from build123d import *

# Parameters (mm, degrees)
SKETCH1_R                = 1.5
SKETCH1_R_2              = 2.5
BOSS_EXTRUDE1_DEPTH      = 20
SKETCH2_W                = 8.1
SKETCH2_H                = 20
SKETCH2_W_2              = 5.2
SKETCH2_W_3              = 5.1
CUT_EXTRUDE1_DEPTH       = 20
CUT_EXTRUDE1_DEPTH_BACK  = 20
CUT_EXTRUDE2_DEPTH       = 9
BOSS_EXTRUDE2_DEPTH      = 11.9
SKETCH5_R                = 3
BOSS_EXTRUDE3_DEPTH      = 5
CUT_EXTRUDE6_DEPTH       = 1
SKETCH13_R               = 2.5
CUT_EXTRUDE7_DEPTH       = 4
BOSS_EXTRUDE4_DEPTH      = 3
CUT_EXTRUDE9_DEPTH       = 3
SKETCH17_W               = 9
SKETCH17_H               = 3.569322199
CUT_EXTRUDE11_DEPTH      = 3
SKETCH18_W               = 5.770974844
SKETCH18_H               = 0.772936936
BOSS_EXTRUDE5_DEPTH      = 6.9
BOSS_EXTRUDE5_DEPTH_BACK = 1
SKETCH19_W               = 5.1
SKETCH19_H               = 16.397725614
CUT_EXTRUDE12_DEPTH      = 0.301495
SKETCH20_W               = 5
SKETCH20_H               = 12.419235667
CUT_EXTRUDE13_DEPTH      = 10
BOSS_EXTRUDE6_DEPTH      = 2
SKETCH23_W               = 4.9
SKETCH23_H               = 6
BOSS_EXTRUDE7_DEPTH      = 4
SKETCH22_R               = 1
CUT_EXTRUDE15_DEPTH      = 8
BOSS_EXTRUDE8_DEPTH      = 2
SKETCH14_R               = 1.5
CUT_EXTRUDE8_DEPTH       = 10.1
CUT_EXTRUDE17_DEPTH      = 8.1
CUT_EXTRUDE17_DEPTH_BACK = 2
CUT_EXTRUDE18_DEPTH      = 2
CUT_EXTRUDE20_DEPTH      = 5.2
SKETCH30_W               = 6.9
SKETCH30_H               = 20
CUT_EXTRUDE21_DEPTH      = 0.283797
CUT_EXTRUDE22_REACH      = 91.699
SKETCH31_W               = 2
SKETCH31_H               = 11.022421386
CUT_EXTRUDE23_DEPTH      = 7


with BuildPart() as part:
    # Sketch1 → Boss-Extrude1 (new body)
    with BuildSketch(Plane(origin=(0, 0, 0), x_dir=(0, 0, -1), z_dir=(1, 0, 0))):
        with BuildLine():
            ThreePointArc((9.765353557, 20.116545894), (0, 32.270117322), (-9.765353557, 20.116545894))
            ThreePointArc((-9.765353557, 20.116545894), (-5.132645827, -18.047253777), (-7.88740095, -56.392382678))
            ThreePointArc((-7.88740095, -56.392382678), (0, -65.729882678), (7.88740095, -56.392382678))
            ThreePointArc((7.88740095, -56.392382678), (5.132645827, -18.047253777), (9.765353557, 20.116545894))
        make_face()
        with Locations((0, 22.270117322)):
            Circle(SKETCH1_R, mode=Mode.SUBTRACT)
        with Locations((0, -57.729882678)):
            Circle(SKETCH1_R_2, mode=Mode.SUBTRACT)
    extrude(amount=BOSS_EXTRUDE1_DEPTH)

    # Sketch2 → Cut-Extrude1 (cut, two sides)
    with BuildSketch(Plane.XY) as cut_extrude1_sk:
        with Locations((4.05, -55.729882678)):
            Rectangle(SKETCH2_W, SKETCH2_H)
        with Locations((17.4, -55.729882678)):
            Rectangle(SKETCH2_W_2, SKETCH2_H)
        with Locations((5.55, 22.270117322)):
            Rectangle(SKETCH2_W_3, SKETCH2_H)
    extrude(amount=CUT_EXTRUDE1_DEPTH, mode=Mode.SUBTRACT)
    extrude(cut_extrude1_sk.sketch, amount=-CUT_EXTRUDE1_DEPTH_BACK, mode=Mode.SUBTRACT)

    # Sketch3 → Cut-Extrude2 (cut)
    with BuildSketch(Plane.ZY.offset(-8.1)):
        with BuildLine():
            Line((8.5, 22.270117322), (8.5, 40.909533312))
            Line((8.5, 40.909533312), (-17.52872033, 40.909533312))
            Line((-17.52872033, 40.909533312), (-17.52872033, 13.770117322))
            Line((-17.52872033, 13.770117322), (0, 13.770117322))
            ThreePointArc((0, 13.770117322), (6.01040764, 16.259709682), (8.5, 22.270117322))
        make_face()
    extrude(amount=-CUT_EXTRUDE2_DEPTH, mode=Mode.SUBTRACT)

    # Sketch4 → Boss-Extrude2 (add, through all)
    with BuildSketch(Plane.ZY.offset(-8.1)):
        Polygon((8.5, 27.537944199), (8.283796844, 12.741558936), (10.283796844, 12.741558936), (10.283796844, 27.537944199), align=None)
    extrude(amount=-BOSS_EXTRUDE2_DEPTH)

    # Sketch5 → Boss-Extrude3 (add)
    with BuildSketch(Plane.ZY.offset(-8.1)):
        with BuildLine():
            Line((8.145156861, 11.968622), (8.447845456, 23.968622))
            Line((8.447845456, 23.968622), (9.854698466, 23.968622))
            Line((9.854698466, 23.968622), (15.022421386, 23.968622))
            ThreePointArc((15.022421386, 23.968622), (21.022421386, 17.968622), (15.022421386, 11.968622))
            Line((15.022421386, 11.968622), (8.145156861, 11.968622))
        make_face()
        with Locations((15.022421386, 17.968622)):
            Circle(SKETCH5_R, mode=Mode.SUBTRACT)
    extrude(amount=-BOSS_EXTRUDE3_DEPTH)

    # Sketch12 → Cut-Extrude6 (cut)
    with BuildSketch(Plane(origin=(13.1, 0, 0), x_dir=(0, 0, -1), z_dir=(1, 0, 0))):
        Polygon((-13.902900694, 14.968622), (-13.902900694, 12.968622), (-15.902900694, 12.968622), (-15.902900694, 14.968622), (-15.902900694, 15.294296094), (-13.902900694, 15.294296094), align=None)
    extrude(amount=-CUT_EXTRUDE6_DEPTH, mode=Mode.SUBTRACT)

    # Sketch13 → Cut-Extrude7 (cut)
    with BuildSketch(Plane.ZY.offset(-17.1)):
        with Locations((0, 22.270117322)):
            Circle(SKETCH13_R)
    extrude(amount=-CUT_EXTRUDE7_DEPTH, mode=Mode.SUBTRACT)

    # Sketch15 → Boss-Extrude4 (add)
    with BuildSketch(Plane.ZY):
        Polygon((10, 22.270117322), (10, 11.968622), (8.145156861, 11.968622), (7.595672539, 11.968622), align=None)
    extrude(amount=-BOSS_EXTRUDE4_DEPTH)

    # Sketch16 → Cut-Extrude9 (cut)
    with BuildSketch(Plane(origin=(20, 0, 0), x_dir=(0, 0, -1), z_dir=(1, 0, 0))):
        with BuildLine():
            Line((-10.283796844, 23.968622), (-9.854698466, 23.968622))
            ThreePointArc((-9.854698466, 23.968622), (-9.349264901, 25.818531871), (-8.5, 27.537944199))
            Line((-8.5, 27.537944199), (-10.283796844, 27.537944199))
            Line((-10.283796844, 27.537944199), (-10.283796844, 23.968622))
        make_face()
    extrude(amount=-CUT_EXTRUDE9_DEPTH, mode=Mode.SUBTRACT)

    # Sketch17 → Cut-Extrude11 (cut)
    with BuildSketch(Plane.XY.offset(10.283796844)):
        with Locations((12.6, 25.7532831)):
            Rectangle(SKETCH17_W, SKETCH17_H)
    extrude(amount=-CUT_EXTRUDE11_DEPTH, mode=Mode.SUBTRACT)

    # Sketch18 → Boss-Extrude5 (add, two sides)
    with BuildSketch(Plane(origin=(13.1, 0, 0), x_dir=(0, 0, -1), z_dir=(1, 0, 0))) as boss_extrude5_sk:
        with Locations((-7.398309422, 12.355090468)):
            Rectangle(SKETCH18_W, SKETCH18_H)
    extrude(amount=BOSS_EXTRUDE5_DEPTH)
    extrude(boss_extrude5_sk.sketch, amount=-BOSS_EXTRUDE5_DEPTH_BACK)

    # Sketch19 → Cut-Extrude12 (cut)
    with BuildSketch(Plane(origin=(0, 12.270117322, 0), x_dir=(1, 0, 0), z_dir=(0, 1, 0))):
        with Locations((5.55, 0)):
            Rectangle(SKETCH19_W, SKETCH19_H)
    extrude(amount=-CUT_EXTRUDE12_DEPTH, mode=Mode.SUBTRACT)

    # Sketch20 → Cut-Extrude13 (cut)
    with BuildSketch(Plane.ZY.offset(-17.1)):
        with Locations((0, 28.479735156)):
            Rectangle(SKETCH20_W, SKETCH20_H)
    extrude(amount=-CUT_EXTRUDE13_DEPTH, mode=Mode.SUBTRACT)

    # Sketch21 → Boss-Extrude6 (add)
    with BuildSketch(Plane.ZY.offset(-17.1)):
        with BuildLine():
            Line((-8.473151119, 13.770117322), (0.278481736, 12.273995678))
            ThreePointArc((0.278481736, 12.273995678), (9.936881703, 21.148341047), (2.5, 31.952575688))
            Line((2.5, 31.952575688), (2.5, 22.270117322))
            ThreePointArc((2.5, 22.270117322), (0, 19.770117322), (-2.5, 22.270117322))
            Line((-2.5, 22.270117322), (-2.5, 31.952575688))
            ThreePointArc((-2.5, 31.952575688), (-8.522477621, 27.501501002), (-9.765353557, 20.116545894))
            ThreePointArc((-9.765353557, 20.116545894), (-9.093560923, 16.948562662), (-8.473151119, 13.770117322))
        make_face()
    extrude(amount=BOSS_EXTRUDE6_DEPTH)

    # Sketch23 → Boss-Extrude7 (add)
    with BuildSketch(Plane.XY.offset(10.283796844)):
        with Locations((17.55, 26.968622)):
            Rectangle(SKETCH23_W, SKETCH23_H)
    extrude(amount=-BOSS_EXTRUDE7_DEPTH)

    # Sketch22 → Cut-Extrude15 (cut)
    with BuildSketch(Plane.XY.offset(10.283796844)):
        with Locations((17.55, 26.870117322)):
            Circle(SKETCH22_R)
    extrude(amount=-CUT_EXTRUDE15_DEPTH, mode=Mode.SUBTRACT)

    # Sketch24 → Boss-Extrude8 (add)
    with BuildSketch(Plane.ZY.offset(-8.1)):
        with BuildLine():
            Line((5.147845456, 19.737443909), (5.147845456, 15.506265819))
            Line((5.147845456, 15.506265819), (8.447845456, 15.506265819))
            Line((8.447845456, 15.506265819), (8.447845456, 23.968622))
            add(Edge.make_bspline(
                [(8.447845456, 23.968622), (5.147845456, 23.968622), (5.147845456, 19.737443909)],
                knots=[3.141592654, 3.141592654, 3.141592654, 4.71238898, 4.71238898, 4.71238898], degree=2, weights=[1, 0.707106781, 1]))
        make_face()
    extrude(amount=-BOSS_EXTRUDE8_DEPTH)

    # Sketch14 → Cut-Extrude8 (cut)
    with BuildSketch(Plane.ZY):
        with Locations((7.532575614, 18.331804915)):
            Circle(SKETCH14_R)
    extrude(amount=-CUT_EXTRUDE8_DEPTH, mode=Mode.SUBTRACT)

    # Sketch25 → Cut-Extrude17 (cut, two sides)
    with BuildSketch(Plane.ZY.offset(-8.1)) as cut_extrude17_sk:
        with BuildLine():
            Line((12, -45.729882678), (8.346153846, -36.960651908))
            ThreePointArc((8.346153846, -36.960651908), (6.973852263, -42.37911752), (2.5, -45.729882678))
            Line((2.5, -45.729882678), (2.5, -53.227383372))
            ThreePointArc((2.5, -53.227383372), (0, -62.879882678), (-2.5, -53.227383372))
            Line((-2.5, -53.227383372), (-2.5, -45.729882678))
            ThreePointArc((-2.5, -45.729882678), (-6.973852263, -42.37911752), (-8.346153846, -36.960651908))
            Line((-8.346153846, -36.960651908), (-12, -45.729882678))
            Line((-12, -45.729882678), (-12, -57.729882678))
            ThreePointArc((-12, -57.729882678), (0, -69.729882678), (12, -57.729882678))
            Line((12, -57.729882678), (12, -45.729882678))
        make_face()
    extrude(amount=CUT_EXTRUDE17_DEPTH, mode=Mode.SUBTRACT)
    extrude(cut_extrude17_sk.sketch, amount=-CUT_EXTRUDE17_DEPTH_BACK, mode=Mode.SUBTRACT)

    # Sketch26 → Cut-Extrude18 (cut)
    with BuildSketch(Plane(origin=(20, 0, 0), x_dir=(0, 0, -1), z_dir=(1, 0, 0))):
        with BuildLine():
            Line((-7.209968303, 15.085404497), (-10.283796844, 15.085404497))
            Line((-10.283796844, 15.085404497), (-10.283796844, 17.085404497))
            Line((-10.283796844, 17.085404497), (-7.209968303, 17.085404497))
            ThreePointArc((-7.209968303, 17.085404497), (-4.010444351, 15.949526558), (-2.243391617, 13.050441039))
            ThreePointArc((-2.243391617, 13.050441039), (0.649659998, -12.257973546), (0.397031114, -37.729953741))
            Line((0.397031114, -37.729953741), (-1.608183929, -37.729953741))
            ThreePointArc((-1.608183929, -37.729953741), (-1.343036313, -12.450773719), (-4.206611504, 12.667092093))
            ThreePointArc((-4.206611504, 12.667092093), (-5.281990934, 14.405678614), (-7.209968303, 15.085404497))
        make_face()
    extrude(amount=-CUT_EXTRUDE18_DEPTH, mode=Mode.SUBTRACT)

    # Sketch29 → Cut-Extrude20 (cut)
    with BuildSketch(Plane(origin=(20, 0, 0), x_dir=(0, 0, -1), z_dir=(1, 0, 0))):
        with BuildLine():
            Line((8, -37.729882678), (8.140336581, -37.729882678))
            Line((8.140336581, -37.729882678), (8.140336581, -45.937498976))
            Line((8.140336581, -45.937498976), (-15.754893946, -45.937498976))
            Line((-15.754893946, -45.937498976), (-15.754893946, -37.729882678))
            Line((-15.754893946, -37.729882678), (-8, -37.729882678))
            ThreePointArc((-8, -37.729882678), (0, -45.729882678), (8, -37.729882678))
        make_face()
    extrude(amount=-CUT_EXTRUDE20_DEPTH, mode=Mode.SUBTRACT)

    # Sketch30 → Cut-Extrude21 (cut)
    with BuildSketch(Plane.XY.offset(10.283796844)):
        with Locations((16.55, 21.968622)):
            Rectangle(SKETCH30_W, SKETCH30_H)
    extrude(amount=-CUT_EXTRUDE21_DEPTH, mode=Mode.SUBTRACT)

    # Sketch31 → Cut-Extrude22 (cut, up to next)
    with BuildSketch(Plane(origin=(0, 23.968622, 0), x_dir=(1, 0, 0), z_dir=(0, 1, 0)), mode=Mode.PRIVATE) as cut_extrude22_sk1:
        with Locations((9.1, -15.511210693)):
            Rectangle(SKETCH31_W, SKETCH31_H)
    cut_extrude22_tool1 = extrude(cut_extrude22_sk1.sketch, amount=-CUT_EXTRUDE22_REACH, mode=Mode.PRIVATE) & part.part
    add(cut_extrude22_tool1.solids().sort_by_distance((9.1, 23.968622, 15.511211))[0], mode=Mode.SUBTRACT)

    # Sketch32 → Cut-Extrude23 (cut)
    with BuildSketch(Plane.ZY.offset(-8.1)):
        Polygon((-8.473151119, 13.770117322), (-8.473151119, 5.401068454), (5.147845456, 15.506265819), align=None)
    extrude(amount=-CUT_EXTRUDE23_DEPTH, mode=Mode.SUBTRACT)


solid = part.part
Check sheet for the modelled part. Datum: model origin and axes. Units: mm. A direction names the side the tool comes from. Give positions to 0.01 mm unless a question says otherwise; leave off trailing zeros. Loops run counter-clockwise (first coordinate to the right, second up) from the corner with the lowest first, then second, coordinate; pieces in that order, holes last. Notation, with made-up numbers: M 53,0 L 78,0 A10 cw 78,16 Z; hole C 14.5,-32 d2. An arc over 180 degrees is marked long. Answer as a JSON object with one key per item and string values. Group by question number.
Q1. Go/stop test with flat-tipped pins: P1, Ø2, axis at y = 8.5, z = 6, coming from the -X side; P2, Ø0.8, axis at x = 12.5, z = 15.5, coming from the +Y side; P3, Ø7, axis at y = 17.97, z = 15.02, coming from the -X side; P4, Ø8, axis at x = 3.5, y = -45, coming from the -Z side. Record where each tip stops, or that it passes through.
Q2. Material ranges on line 1 along Y through (x, z) = (0.75, 0); line 2 along Z through (x, y) = (16.5, -3); line 3 along Y through (x, z) = (11.5, 0), recorded low to high. Write a range as [from, to].
Q3. Access from +Z, -Z, +X, -X, +Y, -Y to the whole of each face (thin tool, end or side, straight path). Record for faces 1 (the flat face through (11.55, 10.79, -1.21)), 2 (the flat face through (9, 18, 10)), 3 (the cylindrical face through (18.01, 25.98, 6.3)), 4 (the flat face through (17, 21, 10)), 5 (the flat face through (19, 17.085, 9)).
Q4. Release check for a two-part mould opening along X. For faces 6 (the flat face through (12.1, 14, 15)), 7 (the flat face through (10.1, -52, 3)), 8 (the flat face through (6, 11.969, 0)), 9 (the flat face through (9, 18, 5.148)) record: released by +X, released by -X, zero draft, split by the parting line, or undercut.
Q5. Cross-section at A-A on y = -4. Record the cut outline in (x, z), then the cut area to 3 significant figures.
Evaluation:
{
 "1": {"P1": "stops at x = 0", "P2": "stops at y = 23.97", "P3": "stops at x = 10.1", "P4": "stops at z = -6.13"},
 "2": {"line 1": "y = [-45.73, 20.77], [23.77, 32.27]", "line 2": "z = [-6.07, 6.07]", "line 3": "y = [-65.73, -60.23], [-55.23, 11.69]"},
 "3": {"face 1": "-Z, +Y", "face 2": "+Z, -X, +Y, -Y", "face 3": "+Z", "face 4": "+Z, +X, +Y, -Y", "face 5": "+Z, +X"},
 "4": {"face 6": "released by +X", "face 7": "released by -X", "face 8": "undercut", "face 9": "undercut"},
 "5": {"outline": "M 0,-5.97 L 20,-5.97 L 20,-0.05 L 18,-0.05 L 18,1.95 L 20,1.95 L 20,5.97 L 0,5.97 Z", "area": "235 mm2"}
}
